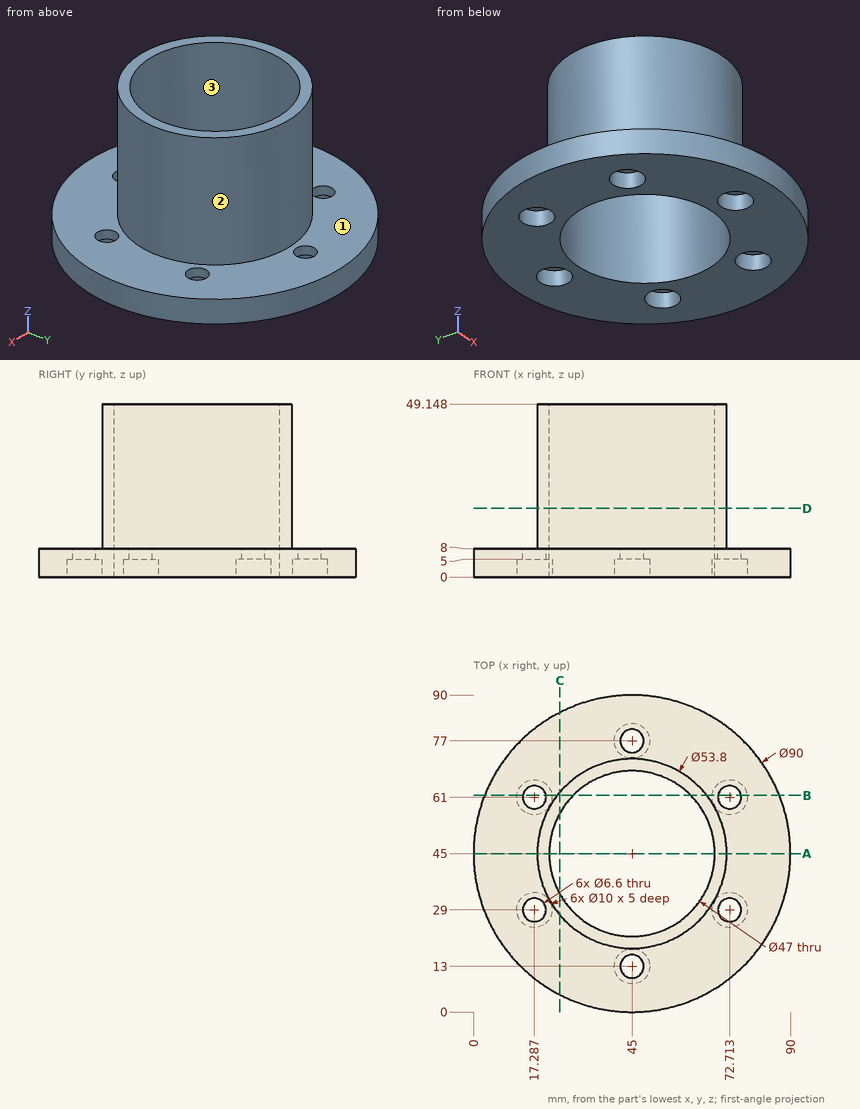
Study the drawing (mm; zero at the part's minimum x, y, z) and answer. Give positions to 0.01 mm unless a question says otherwise; leave off trailing zeros. Write each loop counter-clockwise with the first axis right and the second up, starting at its lowest first coordinate (ties: lowest second). Pieces come first, ordered by that corner, then holes. Notation, with made-up numbers: M 24,18.5 L 64,18.5 A22 ccw 64,52.5 Z; hole C 66,71.25 d10. An arc over 180 degrees is marked long. Put each result on its own line as item: value. Start each with the question number.
1. Consider line 1 along Y through (x, z) = (45, 5.6); line 2 along Z through (x, y) = (67, 63); line 3 along Y through (x, z) = (47.5, 39). Determine where each line is inside the solid, lowest interval first.
2. The part is cut by section C-C, the plane x = 24.5. Give the vertices of the cut face in (y, z), and give its area (3 significant figures).
3. Each of these flat-tipped pins is pushed along its axis until it touches: pin 1 Ø4 at (x, z) = (59, 22.5) entering from +Y (1 decimal); pin 2 Ø3 at (x, y) = (73, 26.5) entering from -Z; pin 3 Ø6 at (x, y) = (72.71, 61) entering from +Z; pin 4 Ø2 at (x, y) = (74.5, 58.5) entering from +Z. Where does it stop, or does it pass through?
4. The part is cut by section B-B, the plane y = 61.5. Give the vertices of the cut face in (x, z) (1 decimal), and give its area (3 significant figures).
5. The part is cut by section A-A, the plane y = 45. Give the vertices of the cut face in (x, z), and give its area (3 significant figures).
6. For a pull along X with two mould halves and no side action, classify the marked faces 1, 2 and 3 as released by +X, released by -X, zero draft, split by the parting line, or undercut.
7. The part is cut by section D-D, the plane z = 19.5. Give the vertices of the cut face in (x, y).
Final values:
1. line 1: y = 0 to 9.7, 16.3 to 21.5, 68.5 to 73.7, 80.3 to 90
1. line 2: z = 0 to 8
1. line 3: y = 18.22 to 21.63, 68.37 to 71.78
2. outline: M 4.94,0 L 33.51,0 L 33.51,49.15 L 27.58,49.15 L 27.58,8 L 4.94,8 Z; M 56.49,0 L 85.06,0 L 85.06,8 L 62.42,8 L 62.42,49.15 L 56.49,49.15 Z
2. area: 945 mm²
3. pin 1: stops at y = 69.1
3. pin 2: stops at z = 5
3. pin 3: passes through
3. pin 4: stops at z = 8
4. outline: M 3.1,0 L 12.3,0 L 12.3,5 L 14,5 L 14,8 L 3.1,8 Z; M 20.5,5 L 22.3,5 L 22.3,0 L 28.3,0 L 28.3,49.1 L 23.8,49.1 L 23.8,8 L 20.5,8 Z; M 61.7,0 L 67.7,0 L 67.7,5 L 69.5,5 L 69.5,8 L 66.2,8 L 66.2,49.1 L 61.7,49.1 Z; M 76,5 L 77.7,5 L 77.7,0 L 86.9,0 L 86.9,8 L 76,8 Z
4. area: 635 mm²
5. outline: M 0,0 L 21.5,0 L 21.5,49.15 L 18.1,49.15 L 18.1,8 L 0,8 Z; M 68.5,0 L 90,0 L 90,8 L 71.9,8 L 71.9,49.15 L 68.5,49.15 Z
5. area: 624 mm²
6. face 1: zero draft
6. face 2: split by the parting line
6. face 3: undercut
7. outline: C 45,45 d53.8; hole C 45,45 d47
